Autodesk Inventor part; units mm, degrees
ref_plane "Work Plane1" through (-38.5, 0, 0) normal (-1, 0, 0) x (0, 0, 1)
ref_plane "YZ Plane" through (0, 0, 0) normal (1, 0, 0) x (0, 1, 0)
ref_plane "XZ Plane" through (0, 0, 0) normal (0, 1, 0) x (-1, 0, 0)
sketch "Sketch1" plane through (0, 0, 0) normal (1, 0, 0) x (0, 1, 0)
  circle A0 centre (0, 0) radius 35
  circle A1 centre (0, 0) radius 8
  dimension "d0" = 70
  dimension "d1" = 16
extrude "Extrusion1" add sketch "Sketch1" along normal blind 7
sketch "Sketch2" plane through (7, 0, 0) normal (1, 0, 0) x (0, 0, -1)
  circle A0 centre (0, 0) radius 23 construction
  point P0 (-23, 0)
  point P1 (-16.2635, -16.2635)
  point P2 (0, -23)
  point P3 (16.2635, -16.2635)
  point P4 (23, 0)
  point P5 (16.2635, 16.2635)
  point P6 (0, 23)
  point P7 (-16.2635, 16.2635)
  dimension "d4" = 46
  dimension "d5" = 0
  dimension "d8" = 360
hole "Hole1" at (7, 0, 23) at (7, -16.2635, 16.2635) at (7, -23, 0) at (7, -16.2635, -16.2635) at (7, 0, -23) at (7, 16.2635, -16.2635) at (7, 23, 0) at (7, 16.2635, 16.2635) direction (-1, 0, 0) diameter 15 depth 5
sketch "Sketch3" plane through (0, 0, 0) normal (-1, 0, 0) x (0, 0, 1)
  circle A0 centre (0, 0) radius 35
  circle A1 centre (0, 0) radius 8
  circle A2 centre (0, 0) radius 9.5
  dimension "d17" = 19
extrude "Extrusion2" add sketch "Sketch3" along normal blind 28 contours A2
sketch "Sketch4" plane through (0, 0, 0) normal (-1, 0, 0) x (0, 0, 1)
  circle A0 centre (0, 0) radius 11
  circle A1 centre (0, 0) radius 9.5
  dimension "d20" = 22
extrude "Extrusion3" add sketch "Sketch4" along normal blind 3
sketch "Sketch5" plane through (-28, 0, 0) normal (-1, 0, 0) x (0, 0, 1)
  circle A0 centre (0, 0) radius 17.5
  circle A1 centre (0, 0) radius 8
  dimension "d23" = 35
extrude "Extrusion4" add sketch "Sketch5" along normal blind 2
sketch "Sketch6" plane through (-30, 0, 0) normal (-1, 0, 0) x (0, 0, 1)
  circle A0 centre (0, 0) radius 17.5
  circle A1 centre (0, 0) radius 8
  circle A2 centre (0, 0) radius 14
  dimension "d26" = 28
  dimension "d27" = 35
extrude "Extrusion5" add sketch "Sketch6" along normal blind 11 contours A0
ref_plane "Work Plane1" through (-38.5, 0, 0) normal (-1, 0, 0) x (0, 0, 1)
sketch "Sketch7" plane through (-38.5, 0, 0) normal (-1, 0, 0) x (0, 0, 1)
  circle A0 centre (0, 0) radius 14
  circle A1 centre (0, 0) radius 14.7
  dimension "d31" = 29.4
extrude "Extrusion6" cut sketch "Sketch7" against normal blind 1.3
sketch "Sketch12" plane through (7, 0, 0) normal (1, 0, 0) x (0, 0, -1)
  circle A0 centre (0, 23) radius 7.5
  circle A1 centre (23, 0) radius 7.5
  circle A2 centre (0, -23) radius 7.5
  circle A3 centre (-23, 0) radius 7.5
  circle A4 centre (-16.2635, -16.2635) radius 7.5
  circle A5 centre (16.2635, -16.2635) radius 7.5
  circle A6 centre (16.2635, 16.2635) radius 7.5
  circle A7 centre (-16.2635, 16.2635) radius 7.5
  circle A8 centre (0, 0) radius 35
  circle A9 centre (0, 0) radius 8
  circle A10 centre (0, 0) radius 28 construction
  line L0 (-16.2635, 16.2635) -> (16.2635, -16.2635) construction
  line L1 (0, 0) -> (0, 23)
  line L2 (0, 0) -> (10.7151, 25.8686)
  line L3 (0, 0) -> (25.8686, 10.7151)
  point P0 (-25.8686, -10.7151)
  point P1 (-10.7151, -25.8686)
  dimension "d41" = 56
  dimension "d42" = 22.5
  dimension "d43" = 45
hole "Hole3" at (7, 25.8686, -10.7151) at (7, 10.7151, -25.8686) at (7, -25.8686, 10.7151) at (7, -10.7151, 25.8686) direction (-1, 0, 0) diameter 4.134 depth 14.2 tip angle 118
sketch "Sketch13" plane through (7, 0, 0) normal (1, 0, 0) x (0, 0, -1)
  circle A0 centre (10.7151, 25.8686) radius 2.067
  circle A1 centre (25.8686, 10.7151) radius 2.067
  line L0 (10.7151, 25.8686) -> (25.8686, 10.7151)
  point P0 (0, 0)
properties part number "P411" material "Aluminum 6061"
The listing builds one solid part. Answer for the finished solid, in the listing's coordinates (mm). A direction names the side the tool comes from. Round coordinates to 2 decimals unless told otherwise and drop trailing zeros. Loops run counter-clockwise (first coordinate to the right, second up) from the corner with the lowest first, then second, coordinate; pieces in that order, holes last.
Q1. Find the intervals of material crossed by line 1 (Z direction, x = 5, y = 0); line 2 (X direction, y = 11.5, z = 7); line 3 (Y direction, x = -39.45, z = 0), in increasing order.
Q2. Given pin 1 Ø2 at (x, y) = (1.5, 6.5) entering from -Z; pin 2 Ø1.5 at (y, z) = (-22, 8) entering from -X; pin 3 Ø9 at (y, z) = (23, 0) entering from +X, each flat-ended and moving along its own axis, determine where each tip first touches the part or whether it passes through.
Q3. Section A-A, the plane x = -14.5 is taken. Determine the outline of the cut face in (y, z).
Q4. Section D-D, the plane y = 21.5 is taken. Determine the outline of the cut face in (x, z), then the cut area to 3 significant figures.
Q5. Which of the six approach directions +Z, -Z, +X, -X, +Y, -Y give full straight-line access (tool end or side, diameter ignored) to faces 1 (the face through (-28, -8, 8)), 2 (the face through (3.45, -11.34, 23.9)), 3 (the face through (2, 0, 23)), 4 (the face through (-33.55, 5.362, 12.932))?
Q6. Section B-B, the plane y = 29.5 is taken. Determine the outline of the cut face in (x, z).
Q7. For a pull along X with two mould halves and no side action, classify faces 5 (the face through (2, -16, -16)), 6 (the face through (-41, 12, -8)), 7 (the face through (0, -8, 8)) as released by +X, released by -X, zero draft, split by the parting line, or undercut.
Q8. Section C-C, the plane z = 20 is taken. Determine the outline of the cut face in (x, y), then the cut area to 3 significant figures.
Completed:
1. line 1: z = -35 to -30.5, -15.5 to -8, 8 to 15.5, 30.5 to 35
1. line 2: x = -30 to -28, 0 to 7
1. line 3: y = -17.5 to -14, 14 to 17.5
2. pin 1: stops at z = -34.57
2. pin 2: stops at x = 0
2. pin 3: stops at x = 2
3. outline: circle Ø19 at (0, 0); hole circle Ø16 at (0, 0)
4. outline: (0, -27.62) - (7, -27.62) - (7, -21.63) - (2, -21.63) - (2, -10.89) - (7, -10.89) - (7, -7.35) - (2, -7.35) - (2, 7.35) - (7, 7.35) - (7, 10.89) - (2, 10.89) - (2, 21.63) - (7, 21.63) - (7, 27.62) - (0, 27.62) - close
4. area: 206 mm2
5. face 1: none
5. face 2: +X, -X
5. face 3: +X
5. face 4: -X
6. outline: (0, -18.83) - (7, -18.83) - (7, -3.74) - (2, -3.74) - (2, 3.74) - (7, 3.74) - (7, 18.83) - (0, 18.83) - close
7. face 5: released by +X
7. face 6: released by -X
7. face 7: undercut
8. outline: (0, -28.72) - (7, -28.72) - (7, -22.77) - (2, -22.77) - (2, -9.76) - (7, -9.76) - (7, -6.87) - (2, -6.87) - (2, 6.87) - (7, 6.87) - (7, 9.76) - (2, 9.76) - (2, 22.77) - (7, 22.77) - (7, 28.72) - (0, 28.72) - close
8. area: 203 mm2
